The listing builds one solid part. Answer for the finished solid, in the listing's coordinates (mm). A direction names the side the tool comes from. Coordinates: 2 decimals unless noted, no trailing zeros. Order: outer loops, then holes, each group sorted by start corner. A loop starts at its lowest first (then second) coordinate and runs counter-clockwise, first axis right, second up. Notation, with made-up numbers: (73.5, 12) -> (114.5, 12) arc R18 ccw to (114.5, 45) -> close; hole circle Ø8 at (10, 62). An arc over 180 degrees is marked (long way). Return JSON: item names as keys, results as strings.
from build123d import *

# Parameters (mm, degrees)
SM_BASE_FLANGE_1_DEPTH = 7
CUT_EXTRUDE_1_DEPTH    = 25.859605789
SKETCH_4_W             = 2.7366
SKETCH_4_H             = 15
CUT_EXTRUDE_2_DEPTH    = 4
FILLET_1_R             = 5
SKETCH_5_R             = 2.6
CUT_EXTRUDE_3_DEPTH    = 25.454038521


# Sheet-metal steps are written as plain solids
with BuildPart() as part:
    # Sketch 1 → 基体-法兰1 (new, symmetric)
    with BuildSketch(Plane(origin=(0, 0, 0), x_dir=(0, 0, -1), z_dir=(1, 0, 0))):
        with BuildLine():
            Line((-20, 0), (-2.7366, 0))
            ThreePointArc((-2.7366, 0), (-0.801531583, 0.801531583), (0, 2.7366))
            Line((0, 2.7366), (0, 15))
            Line((0, 15), (-2, 15))
            Line((-2, 15), (-2, 2.7366))
            ThreePointArc((-2, 2.7366), (-2.215745145, 2.215745145), (-2.7366, 2))
            Line((-2.7366, 2), (-20, 2))
            Line((-20, 2), (-20, 0))
        make_face()
    extrude(amount=SM_BASE_FLANGE_1_DEPTH, both=True)

    # 草图3 → 切除-拉伸1 (cut, through all)
    with BuildSketch(Plane(origin=(0, 2, 0), x_dir=(1, 0, 0), z_dir=(0, 1, 0))):
        with BuildLine():
            Line((-3, -11.75), (3, -11.75))
            ThreePointArc((3, -11.75), (5.25, -14), (3, -16.25))
            Line((3, -16.25), (-3, -16.25))
            ThreePointArc((-3, -16.25), (-5.25, -14), (-3, -11.75))
        make_face()
    extrude(amount=-CUT_EXTRUDE_1_DEPTH, mode=Mode.SUBTRACT)

    # 草图4 → 切除-拉伸2 (cut)
    with BuildSketch(Plane.ZY.offset(-7)):
        with Locations((1.3683, 7.5)):
            Rectangle(SKETCH_4_W, SKETCH_4_H)
    extrude(amount=CUT_EXTRUDE_2_DEPTH, mode=Mode.SUBTRACT)

    # 圆角1
    fillet_1_edges = [part.edges().sort_by_distance(p)[0] for p in [
        (-7, 1, 20),
        (7, 1, 20),
        (3, 15, 1),
        (-7, 15, 1),
    ]]
    fillet(fillet_1_edges, radius=FILLET_1_R - 0.0001)  # a hair under: the kernel refuses the full size

    # 草图5 → 切除-拉伸3 (cut, through all)
    with BuildSketch(Plane.XY.offset(2)):
        with Locations((-2, 10)):
            Circle(SKETCH_5_R)
    extrude(amount=-CUT_EXTRUDE_3_DEPTH, mode=Mode.SUBTRACT)


solid = part.part
1. Determine the mould class of faces 6 (the face through (-2.56, 7.46, 1.01)), 7 (the face through (0, 1, 11.75)), 8 (the face through (0, 1, 20)), 9 (the face through (-6, 13, 1)) for opening direction X: pulls with the +X half, pulls with the -X half, needs draft (parallel to the pull), parting line crosses it, or undercut.
Answer block:
{"face 6": "undercut", "face 7": "undercut", "face 8": "needs draft", "face 9": "pulls with the -X half"}
2. The part is cut by section A-A on z = 14.5. Give the vertices of the cut face in (x, y), and give its area (3 significant figures).
Answer block:
{"outline": "(-7, 0) -> (-5.19, 0) -> (-5.19, 2) -> (-7, 2) -> close; (5.19, 0) -> (7, 0) -> (7, 2) -> (5.19, 2) -> close", "area": "7.23 mm2"}
3. The part is cut by section C-C on x = -5. Give the vertices of the cut face in (y, z).
Answer block:
{"outline": "(0, 2.74) arc R2.74 ccw to (2.74, 0) -> (14, 0) -> (14, 2) -> (2.74, 2) arc R0.74 cw to (2, 2.74) -> (2, 12.97) -> (0, 12.97) -> close; (0, 15.03) -> (2, 15.03) -> (2, 19) -> (0, 19) -> close"}
4. The part is cut by section B-B on y = 11.25. Give the vertices of the cut face in (x, z).
Answer block:
{"outline": "(-6.84, 0) -> (-4.28, 0) -> (-4.28, 2) -> (-6.84, 2) -> close; (0.28, 0) -> (2.84, 0) -> (2.84, 2) -> (0.28, 2) -> close"}
5. Each of these flat-tipped pins is pushed along its axis until it touches: pin 1 Ø7 at (x, z) = (2.5, 15.5) entering from +Y; pin 2 Ø3 at (x, y) = (-2, 7.5) entering from +Z; pin 3 Ø1 at (x, y) = (5.5, 1.5) entering from -Z. Where does it stop, or does it pass through?
Answer block:
{"pin 1": "stops at y = 2", "pin 2": "stops at z = 2", "pin 3": "stops at z = 2.74"}
6. Consider line 1 (Z direction, x = -5.75, y = 11.5); line 2 (X direction, y = 5, z = 1). Determine where each line is inside the solid, lowest interval first. Write a range as from..to.
Answer block:
{"line 1": "z = 0..2", "line 2": "x = -7..3"}
7. For faces 1 (the face through (-7, 1.7, 5.3)), 2 (the face through (0, 2, 11)), 3 (the face through (-5.25, 1.01, 14.05)), 4 (the face through (1, 14, 1)), 5 (the face through (3, 5, 1)), determine the directions among +Z, -Z, +X, -X, +Y, -Y from which every point of the face is accessible in a straight line to the end or side of a thin tool.
Answer block:
{"face 1": "+Z, -Z, -X, +Y, -Y", "face 2": "+Z, +X, -X, +Y", "face 3": "+Y, -Y", "face 4": "+Z, -Z, +X, +Y", "face 5": "-Z, +X, +Y, -Y"}
